from build123d import *

# Parameters (mm, degrees)
SKETCH2_R                      = 30
BOSS_EXTRUDE1_DEPTH            = 20
CUT_EXTRUDE2_DEPTH             = 47.904157598
M3_CLEARANCE_HOLE1_D           = 3.4
M3_CLEARANCE_HOLE1_CSINK_D     = 3.45
M3_CLEARANCE_HOLE1_CSINK_ANGLE = 90
CUT_EXTRUDE3_DEPTH             = 47.904157598


with BuildPart() as part:
    # Sketch2 → Boss-Extrude1 (new body)
    with BuildSketch(Plane(origin=(0, 0, 0), x_dir=(1, 0, 0), z_dir=(0, 1, 0))):
        with Locations(Location((0, 0, 0), (0, 0, 270))):
            Circle(SKETCH2_R)
    extrude(amount=BOSS_EXTRUDE1_DEPTH)

    # Sketch3 → Cut-Extrude2 (cut, through all)
    with BuildSketch(Plane(origin=(0, 20, 0), x_dir=(1, 0, 0), z_dir=(0, 1, 0))):
        with BuildLine():
            ThreePointArc((0, -17.5), (17.5, 0), (0, 17.5))
            Line((0, 17.5), (-2, 17.5))
            Line((-2, 17.5), (-2, 9.06190379))
            Line((-2, 9.06190379), (-2, 6.812488532))
            ThreePointArc((-2, 6.812488532), (-7.1, 0), (-2, -6.812488532))
            Line((-2, -6.812488532), (-2, -9.06190379))
            Line((-2, -9.06190379), (-2, -17.5))
            Line((-2, -17.5), (0, -17.5))
        make_face()
    extrude(amount=-CUT_EXTRUDE2_DEPTH, mode=Mode.SUBTRACT)

    # M3 Clearance Hole1 (through all)
    with Locations(Plane(origin=(0, 0, 0), x_dir=(-1, 0, 0), z_dir=(0, -1, 0))):
        with Locations((0, 23.75), (-23.75, 0), (0, -23.75)):
            CounterSinkHole(M3_CLEARANCE_HOLE1_D / 2, M3_CLEARANCE_HOLE1_CSINK_D / 2, counter_sink_angle=M3_CLEARANCE_HOLE1_CSINK_ANGLE)

    # Sketch6 → Cut-Extrude3 (cut, through all)
    with BuildSketch(Plane(origin=(0, 20, 0), x_dir=(1, 0, 0), z_dir=(0, 1, 0))):
        with BuildLine():
            Line((-24.366985862, 17.5), (-2, 17.5))
            Line((-2, 17.5), (-2, -17.5))
            Line((-2, -17.5), (-24.366985862, -17.5))
            ThreePointArc((-24.366985862, -17.5), (-30, 0), (-24.366985862, 17.5))
        make_face()
    extrude(amount=-CUT_EXTRUDE3_DEPTH, mode=Mode.SUBTRACT)

    # Sketch8 → CBORE for M3 SHCS1 (revolve, cut)
    with BuildSketch(Plane(origin=(-12.046985862, 10, 30), x_dir=(0, -1, 0), z_dir=(1, 0, 0))):
        Polygon((0, 0), (0, 12.5), (1.7, 12.5), (1.7, 7), (3.25, 7), (3.25, 0.025), (3.275, 0), align=None)
    cbore_for_m3_shcs1 = revolve(axis=Axis((-12.046985862, 10, 36.35), (0, 0, -1)), mode=Mode.SUBTRACT)

    # Mirror1: CBORE for M3 SHCS1 across plane
    add(cbore_for_m3_shcs1.mirror(Plane.XY), mode=Mode.SUBTRACT)


solid = part.part
Geometry check sheet. Reference: the model listing, model coordinates, mm. A direction names the side the tool comes from. Round coordinates to 2 decimals unless told otherwise and drop trailing zeros. Loops run counter-clockwise (first coordinate to the right, second up) from the corner with the lowest first, then second, coordinate; pieces in that order, holes last. Notation, with made-up numbers: (66, 85) -> (115, 85) arc R35 ccw to (115, 119) -> close; hole circle Ø2 at (73, 38). An arc over 180 degrees is marked (long way). Answer as a JSON object with one key per item and string values. Group by question number.
Item 1: Thickness scan on line 1 along X through (y, z) = (12, 24.5); line 2 along Z through (x, y) = (7, 7.5); line 3 along Z through (x, y) = (-10, 11.25). Record the ranges inside material, lowest first.
Item 2: Cross-section at D-D, the plane x = -17.5. Record the cut outline in (y, z).
Item 3: Release check for a two-part mould opening along X. For faces 4 (the face through (17.496, 10.14, 0.385)), 5 (the face through (-0.221, 10.152, 22.064)), 6 (the face through (21, 0, 0)) record: pulls with the +X half, pulls with the -X half, needs draft (parallel to the pull), parting line crosses it, or undercut.
Item 4: Cross-section at B-B, the plane y = 5.25. Record the cut outline in (x, z), plus the area to 3 significant figures.
Item 5: Cross-section at A-A, the plane z = 0. Record the cut outline in (x, y) (3 decimals).
Item 6: Cross-section at C-C, the plane z = -23.75. Record the cut outline in (x, y) (3 decimals), plus the area to 3 significant figures.
Item 7: Set-up check for faces 1 (the face through (-12, 8, -17.5)), 2 (the face through (-8.874, 10.705, 25.249)), 3 (the face through (-8.874, 10.705, -25.249)): record each of +Z, -Z, +X, -X, +Y, -Y from which the full face is reachable in a straight line by a thin tool's end or side.
Item 8: Depth check by flat-ended pin: pin 1 Ø1 at (x, y) = (12.5, 15.5) entering from -Z; pin 2 Ø10.5 at (x, y) = (-12.05, 10) entering from -Z; pin 3 Ø2 at (x, y) = (-8.5, 10) entering from -Z; pin 4 Ø5.5 at (x, z) = (0, 23.75) entering from +Y. Enter the tip coordinate at first touch or a pass-through.
Determined:
{
 "1": {"line 1": "x = -17.31 to -14.61, -9.49 to -1.53, 1.53 to 17.31", "line 2": "z = -29.17 to -16.04, 16.04 to 29.17", "line 3": "z = -23 to -17.5, 17.5 to 23"},
 "2": {"outline": "(0, -24.37) -> (20, -24.37) -> (20, -17.5) -> (0, -17.5) -> close; (0, 17.5) -> (20, 17.5) -> (20, 24.37) -> (0, 24.37) -> close"},
 "3": {"face 4": "pulls with the -X half", "face 5": "undercut", "face 6": "needs draft"},
 "4": {"outline": "(-24.37, -17.5) arc R30 ccw (long way) to (-24.37, 17.5) -> (0, 17.5) arc R17.5 cw to (0, -17.5) -> close; hole circle Ø3.4 at (0, -23.75); hole circle Ø3.4 at (0, 23.75); hole circle Ø3.4 at (23.75, 0)", "area": "1,330 mm²"},
 "5": {"outline": "(17.5, 0) -> (22.025, 0) -> (22.05, 0.025) -> (22.05, 20) -> (17.5, 20) -> close; (25.45, 0.025) -> (25.475, 0) -> (30, 0) -> (30, 20) -> (25.45, 20) -> close"},
 "6": {"outline": "(-18.329, 0) -> (-1.725, 0) -> (-1.7, 0.025) -> (-1.7, 20) -> (-18.329, 20) -> close; (1.7, 0.025) -> (1.725, 0) -> (18.329, 0) -> (18.329, 20) -> (1.7, 20) -> close; hole circle Ø6.5 at (-12.047, 10)", "area": "632 mm²"},
 "7": {"face 1": "-X, +Y, -Y", "face 2": "+Z", "face 3": "-Z"},
 "8": {"pin 1": "stops at z = -27.5", "pin 2": "stops at z = -29.22", "pin 3": "stops at z = -29.05", "pin 4": "stops at y = 20"}
}
